from build123d import *

# Parameters (mm, degrees)
F0_R     = 15
F1_DEPTH = 2
F2_R     = 11.125
F2_R_2   = 10
F3_DEPTH = 8
F4_SIZE2 = 6.8580313817
F4_SIZE  = 0.6


with BuildPart() as f1:
    # F0 (on Top) → F1 (new body)
    with BuildSketch(Plane.XY):
        Circle(F0_R)
    extrude(amount=F1_DEPTH)

    # F2 (on face) → F3 (join)
    with BuildSketch(Plane(origin=(0, 0, 0), x_dir=(1, 0, 0), z_dir=(0, 0, -1))):
        Circle(F2_R)
        Circle(F2_R_2, mode=Mode.SUBTRACT)
    extrude(amount=F3_DEPTH)

    # F4
    f4_edges = [f1.edges().sort_by_distance(p)[0] for p in [
        (-11.125, 0, -8),
    ]]
    f4_side = f1.faces().sort_by_distance((-10.810337, 0, -8))[0]
    chamfer(f4_edges, length=F4_SIZE, length2=F4_SIZE2, reference=f4_side)

    # F5 (on Front) → F6 (revolve)
    with BuildSketch(Plane.XZ):
        with BuildLine():
            Line((0, 4.9190075645), (0, 2))
            Line((0, 2), (15, 2))
            ThreePointArc((15, 2), (7.6406904983, 4.1824746645), (0, 4.9190075645))
        make_face()
    revolve(axis=Axis((0, 0, 3.4595037823), (0, 0, 1)))


solid = f1.part
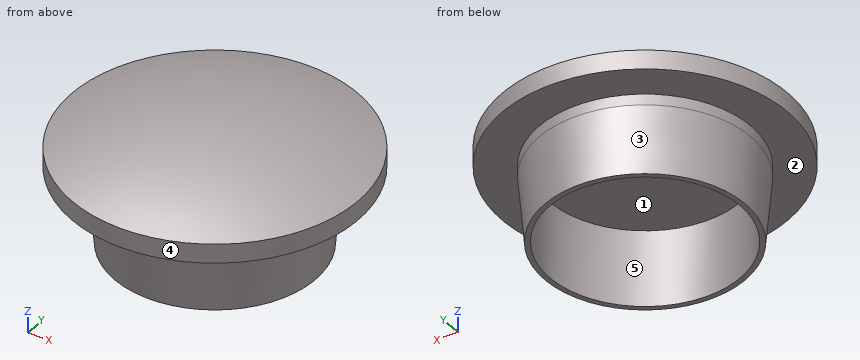
Verification items for the finished model (mm, model axes). Face numbers are marked on the shaded views. A direction names the side the tool comes from. Coordinates: 2 decimals unless noted, no trailing zeros. Order: outer loops, then holes, each group sorted by start corner. A loop starts at its lowest first (then second) coordinate and runs counter-clockwise, first axis right, second up. Notation, with made-up numbers: M 38,-20.75 L 95,-20.75 A14 cw 95,-11.75 Z; hole C 79,89 d3. An arc over 180 degrees is marked long. One line per item, written item: value. Start each with the question number.
Item 1: Sectioned sample at A-A (x = 0). Enter the section's corners in (y, z) (3 decimals), then the cut area to 3 significant figures.
Item 2: Mould release check, pull along Y, two halves, no side actions. Record for the marked faces 1, 2 and 3: released by +Y, released by -Y, zero draft, split by the parting line, or undercut.
Item 3: Gauge pin test, flat ends, axial feed: pin 1 (5 mm diameter, centred on x = 6.5, z = -0.5, fed in from +Y); pin 2 (1.5 mm diameter, centred on y = 11.5, z = -0.5, fed in from -X); pin 3 (4 mm diameter, centred on y = -4, z = 3.5, fed in from -X). Record the tip position at first contact, or that the pin passes through.
Item 4: Scan lines: probe 1 along X at (y, z) = (0, -4.5); probe 2 along X at (y, z) = (0, -5.75); probe 3 along Y at (x, z) = (0, -2.25). Record each from-to range of solid material in increasing order.
Item 5: Sectioned sample at D-D (z = 0.5). Enter the section's corners in (x, y), then the cut area to 3 significant figures.
Item 6: Access from +Z, -Z, +X, -X, +Y, -Y to the whole of each face (thin tool, end or side, straight path). Record for the marked faces 4 and 5.
Conclusion:
1. outline: M -15,0 L -11.125,0 L -11.125,-1.142 L -10.525,-8 L -10,-8 L -10,0 L 10,0 L 10,-8 L 10.525,-8 L 11.125,-1.142 L 11.125,0 L 15,0 L 15,2 A40 ccw -15,2 Z
1. area: 133 mm^2
2. face 1: undercut
2. face 2: zero draft
2. face 3: split by the parting line
3. pin 1: stops at y = 14.44
3. pin 2: stops at x = -10.26
3. pin 3: stops at x = -14.76
4. probe 1: x = -10.83 to -10, 10 to 10.83
4. probe 2: x = -10.72 to -10, 10 to 10.72
4. probe 3: y = -11.03 to -10, 10 to 11.03
5. outline: C 0,0 d30
5. area: 707 mm^2
6. face 4: +Z, -Z
6. face 5: -Z
